Here's how the part is built. I have some questions about the finished solid (model axes, mm). Give positions to 0.01 mm unless a question says otherwise; leave off trailing zeros. Loops run counter-clockwise (first coordinate to the right, second up) from the corner with the lowest first, then second, coordinate; pieces in that order, holes last.
Q1. Suppose I cut it at A-A (x = -51). List the corners of the cut face in (y, z) for me, and give its area (3 significant figures).
Q2. Suppose I cut it at C-C (x = -26.5). List the corners of the cut face in (y, z) for me.
Q3. Suppose I cut it at B-B (y = 2.25). List the corners of the cut face in (x, z) for me, and give its area (3 significant figures).
Q4. I'm going to push flat-ended pins straight in: P1, Ø8, axis at x = -52.5, z = -70, coming from the -Y side; P2, Ø1.5, axis at y = 6, z = -57, coming from the +X side; P3, Ø12, axis at x = -31.5, z = -34, coming from the +Y side; P4, Ø1.5, axis at x = -52, y = 5, coming from the +Z side. Where does each tip first touch, or does it pass through?
Q5. I need wall thicknesses on probe 1 along Z at (x, y) = (-14, 2.25); probe 2 along Z at (x, y) = (-46, 2.25); probe 3 along X at (y, z) = (2, -159). Which ranges of each line are inside material? Lowest first, please.
Q6. Thinking about a two-plate mould opening in Z: for faces 1 (the face through (-64.304, 3.451, -94.415)), 2 (the face through (-61.7, 6, -97.8)), 3 (the face through (-61, 5, -103)), 4 (the face through (0, 3, -2)), which applies, pulls with the +Z half, pulls with the -Z half, needs draft (parallel to the pull), parting line crosses it, or undercut?
Q7. Suppose I cut it at D-D (z = -34). List the corners of the cut face in (x, y) for me, and give its area (3 significant figures).
Autodesk Inventor part; units mm, degrees
ref_plane "YZ Plane" through (0, 0, 0) normal (1, 0, 0) x (0, 1, 0)
ref_plane "XZ Plane" through (0, 0, 0) normal (0, 1, 0) x (-1, 0, 0)
ref_plane "XY Plane" through (0, 0, 0) normal (0, 0, 1) x (1, 0, 0)
sketch "Эскиз1" plane through (0, 0, 0) normal (0, 1, 0) x (-1, 0, 0)
  line L0 (0, 0) -> (0, -192.264)
  arc A0 (0, -192.264) -> (0, 0) centre (-39.6817, -96.132) ccw
  line L1 (0, 0) -> (0, -5)
  line L2 (0, -192.264) -> (0, -187.264)
  arc A1 (0, -187.264) -> (0, -5) centre (-39.6817, -96.132) ccw
  dimension "d0" = 192.264
  dimension "d1" = 104
  dimension "d2" = 5
  dimension "d3" = 5
  dimension "d4" = 99.3966
extrude "Выдавливание1" add sketch "Эскиз1" along normal blind 7 contours A0 L0 A1
sketch "Эскиз2" plane through (0, 7, 0) normal (0, 1, 0) x (1, 0, 0)
  arc A0 (0, 187.264) -> (0, 5) centre (39.6817, 96.132) ccw
  arc A1 (-0.7985, 189.0977) -> (-0.7985, 3.1663) centre (39.6817, 96.132) ccw
  line L0 (-0.7985, 3.1663) -> (0, 2.8227)
  line L1 (-0.7985, 189.0977) -> (0, 189.4413)
  line L2 (0, 0) -> (0, 5)
  line L3 (0, 2.8227) -> (0, 5)
  line L4 (0, 189.4413) -> (0, 187.264)
  arc A2 (0, 187.264) -> (0, 5) centre (39.6817, 96.132) ccw
  dimension "d8" = 2
extrude "Выдавливание2" cut sketch "Эскиз2" against normal blind 2
sketch "Эскиз3" plane through (0, 0, 0) normal (1, 0, 0) x (0, 1, 0)
  line L0 (5, -91.132) -> (0, -91.132)
  line L1 (0, -91.132) -> (0, -101.132)
  line L2 (0, -101.132) -> (5, -101.132)
  line L3 (5, -101.132) -> (5, -91.132)
  line L4 (0, -187.264) -> (5, -187.264)
  point P0 (2.5, -187.264)
  point P1 (2.5, -101.132)
  dimension "d11" = 5
  dimension "d12" = 10
  dimension "d13" = 86.132
Solutions:
1. outline: (0, -147.05) - (7, -147.05) - (7, -141.5) - (5, -141.5) - (5, -136.83) - (0, -136.83) - close; (0, -55.43) - (5, -55.43) - (5, -50.77) - (7, -50.77) - (7, -45.21) - (0, -45.21) - close
1. area: 124 mm2
2. outline: (0, -176.36) - (7, -176.36) - (7, -172.95) - (5, -172.95) - (5, -170.29) - (0, -170.29) - close; (0, -21.97) - (5, -21.97) - (5, -19.31) - (7, -19.31) - (7, -15.91) - (0, -15.91) - close
3. outline: (0, -192.26) - (0, -187.26) arc R99.4 cw to (0, -5) - (0, 0) arc R104 ccw to start
3. area: 1,100 mm2
4. P1: stops at y = 0
4. P2: stops at x = -53.54
4. P3: stops at y = 5
4. P4: stops at z = -45.66
5. probe 1: z = -185.21 to -179.79, -12.48 to -7.06
5. probe 2: z = -155.08 to -146.51, -45.75 to -37.19
5. probe 3: x = -43.17 to -37.31
6. face 1: parting line crosses it
6. face 2: undercut
6. face 3: undercut
6. face 4: needs draft
7. outline: (-43.72, 0) - (-37.9, 0) - (-37.9, 5) - (-40.45, 5) - (-40.45, 7) - (-43.72, 7) - close
7. area: 35.6 mm2
